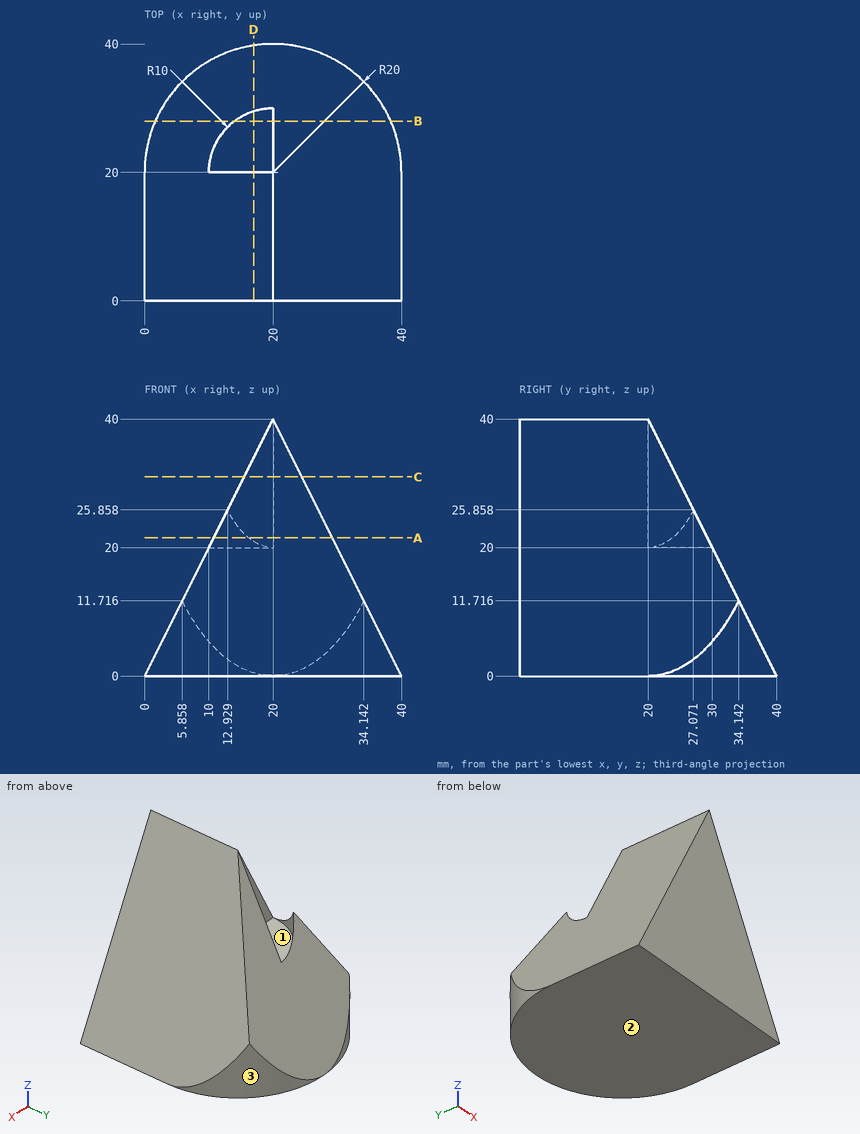
Geometry check sheet. Reference: drawing and pictorial views, mm from the part's lowest x, y, z. Coordinates: 2 decimals unless noted, no trailing zeros. Loops run counter-clockwise (first coordinate to the right, second up) from the corner with the lowest first, then second, coordinate; pieces in that order, holes last.
1) Sectioned sample at A-A (z = 21.5). Record the boundary of the cut face in (x, y).
2) Gauge pin test, flat ends, axial feed: pin 1 (6 mm diameter, centred on y = 8.5, z = 13.5, fed in from +X); pin 2 (5 mm diameter, centred on y = 25.5, z = 32, fed in from -X); pin 3 (3 mm diameter, centred on x = 23.5, y = 20, fed in from +Z). Record the tip position at first contact, or that the pin passes through.
3) Sectioned sample at C-C (z = 31). Record the boundary of the cut face in (x, y).
4) Material ranges on probe 1 along Z at (x, y) = (35, 4.5); probe 2 along Y at (x, z) = (27, 19); probe 3 along Z at (x, y) = (33.5, 21), recorded low to high.
5) Sectioned sample at D-D (x = 17). Record the boundary of the cut face in (y, z), and give its area (3 significant figures).
6) Release check for a two-part mould opening along X. For the marked faces 1, 2 and 3 record: released by +X, released by -X, zero draft, split by the parting line, or undercut.
7) Sectioned sample at B-B (y = 28). Record the boundary of the cut face in (x, z), and give its area (3 significant figures).
Check sheet entries:
1. outline: (10.75, 0) - (29.25, 0) - (29.25, 29.25) - (20, 29.25) - (20, 20) - (10.75, 20) - close; (10.75, 23.8) arc R10 cw to (16.2, 29.25) - (10.75, 29.25) - close
2. pin 1: stops at x = 34.75
2. pin 2: stops at x = 20
2. pin 3: stops at z = 36
3. outline: (15.5, 0) - (24.5, 0) - (24.5, 24.5) - (20, 24.5) - (20, 20) - (15.5, 20) - close
4. probe 1: z = 0 to 10
4. probe 2: y = 0 to 30.5
4. probe 3: z = 0 to 13
5. outline: (0, 0) - (39.77, 0) - (39.77, 0.45) - (29.54, 20.92) - (29.54, 20) - (20, 20) - (20, 34) - (0, 34) - close
5. area: 980 mm2
6. face 1: undercut
6. face 2: zero draft
6. face 3: released by +X
7. outline: (1.67, 0) - (38.33, 0) - (38.33, 3.34) - (28, 24) - (20, 24) - (20, 20) - (14, 20) - (14, 24) - (12, 24) - (1.67, 3.34) - close
7. area: 642 mm2
